Work out the finished part from the listing and answer in its coordinate system (mm). Round coordinates to 2 decimals unless told otherwise and drop trailing zeros. Loops run counter-clockwise (first coordinate to the right, second up) from the corner with the lowest first, then second, coordinate; pieces in that order, holes last. Notation, with made-up numbers: (10.25, 65) - (35.25, 65) arc R16 cw to (35.25, 80) - close; hole circle Ø6 at (64.5, 55). An arc over 180 degrees is marked (long way). Answer as CSV lines item,"result". Start each with the question number.
Q1. Section D-D on x = 39.5 is taken. Write down the section's boundary in (y, z).
Q2. Section C-C on z = 0.2 is taken. Write down the section's boundary in (x, y), then the cut area to 3 significant figures.
Q3. Section A-A on y = 0 is taken. Write down the section's boundary in (x, z).
Q4. The mould has two halves that part along Y. Classify faces 1 (the face through (1, 2, -1.588)), 2 (the face through (-30.757, 1.021, -0.022)), 3 (the face through (42.15, -9.49, 0.02)), 4 (the face through (-1, 16, 0)): +Y half, -Y half, draft (parallel to the pull), parting line (faces both ways), or undercut.
Q5. Straight lines are drawn through the part: L1, parallel to Y at x = 34, z = 0.8; L2, parallel to X at y = -1.5, z = -0.7; L3, parallel to Y at x = -36, z = -1. For each, find the intervals that lie inside material, in ascending order. Write a range as [from, to].
Q6. Section B-B on x = -34 is taken. Write down the section's boundary in (y, z), then the cut area to 3 significant figures.
```python
from build123d import *

# Parameters (mm, degrees)
SKETCH1_R           = 3.4
BOSS_EXTRUDE1_DEPTH = 1.5875
FILLET1_R           = 10
FILLET2_R           = 1


with BuildPart() as part:
    # Sketch1 → Boss-Extrude1 (new, symmetric)
    with BuildSketch(Plane.XY):
        Polygon((-45, 12.499999995), (-45, 15.999999995), (45, 15.999999995), (45, 12.499999995), (45, -12.499999995), (-45, -12.499999995), align=None)
        with Locations((34, 0)):
            Circle(SKETCH1_R, mode=Mode.SUBTRACT)
        with Locations((-34, 0)):
            Circle(SKETCH1_R, mode=Mode.SUBTRACT)
    extrude(amount=BOSS_EXTRUDE1_DEPTH, both=True)

    # Fillet1
    fillet1_edges = [part.edges().sort_by_distance(p)[0] for p in [
        (45, -12.499999995, 0),
        (-45, -12.499999995, 0),
    ]]
    fillet(fillet1_edges, radius=FILLET1_R)

    # Fillet2
    fillet2_edges = [part.edges().sort_by_distance(p)[0] for p in [
        (-45, 15.999999995, 0),
        (45, 15.999999995, 0),
    ]]
    fillet(fillet2_edges, radius=FILLET2_R)


solid = part.part
```
Findings:
1,outline,"(-11.43, -1.59) - (16, -1.59) - (16, 1.59) - (-11.43, 1.59) - close"
2,outline,"(-45, -2.5) arc R10 ccw to (-35, -12.5) - (35, -12.5) arc R10 ccw to (45, -2.5) - (45, 15) arc R1 ccw to (44, 16) - (-44, 16) arc R1 ccw to (-45, 15) - close; hole circle Ø6.8 at (-34, 0); hole circle Ø6.8 at (34, 0)"
2,area,"2,450 mm^2"
3,outline,"(-45, -1.59) - (-37.4, -1.59) - (-37.4, 1.59) - (-45, 1.59) - close; (-30.6, -1.59) - (30.6, -1.59) - (30.6, 1.59) - (-30.6, 1.59) - close; (37.4, -1.59) - (45, -1.59) - (45, 1.59) - (37.4, 1.59) - close"
4,face 1,"draft"
4,face 2,"undercut"
4,face 3,"-Y half"
4,face 4,"+Y half"
5,L1,"y = [-12.5, -3.4], [3.4, 16]"
5,L2,"x = [-45, -37.05], [-30.95, 30.95], [37.05, 45]"
5,L3,"y = [-12.45, -2.75], [2.75, 16]"
6,outline,"(-12.5, -1.59) - (-3.4, -1.59) - (-3.4, 1.59) - (-12.5, 1.59) - close; (3.4, -1.59) - (16, -1.59) - (16, 1.59) - (3.4, 1.59) - close"
6,area,"68.9 mm^2"
